```python
from build123d import *

# Parameters (mm, degrees)
SKETCH_1_W                       = 60
SKETCH_1_H                       = 1.5
SM_BASE_FLANGE_1_DEPTH           = 150
SM_EDGE_FLANGE_1_DEPTH           = 150
SM_EDGE_FLANGE_1_2_DEPTH         = 150
SM_EDGE_FLANGE_2_STRIP_W         = 7.4732
SM_EDGE_FLANGE_2_STRIP_H         = 1.5
SM_EDGE_FLANGE_2_STRIP_CUT_DEPTH = 150
SM_EDGE_FLANGE_2_DEPTH           = 150
SKETCH_12_R                      = 2.1
CUT_EXTRUDE_1_DEPTH              = 10
SM_EDGE_FLANGE_3_DEPTH           = 150
SM_EDGE_FLANGE_3_2_DEPTH         = 150
SKETCH_16_R                      = 2.1
CUT_EXTRUDE_2_DEPTH              = 20


# Read off the part's stored shape, not the designer's step: 边线-法兰1, 边线-法兰3
# Sheet-metal steps are written as plain solids
with BuildPart() as part:
    # Sketch 1 → 基体-法兰1 (new body)
    with BuildSketch(Plane.XY):
        with Locations((30, -0.75)):
            Rectangle(SKETCH_1_W, SKETCH_1_H)
    extrude(amount=SM_BASE_FLANGE_1_DEPTH)

    # 边线-法兰1 outline → 边线-法兰1 (cut)
    with BuildSketch(Plane.XY):
        with BuildLine():
            ThreePointArc((54.107469813, 0), (54.399404694, -0.019134423), (54.686344489, -0.076210297))
            Line((54.686344489, -0.076210297), (60, -1.5))
            Line((60, -1.5), (60, 0))
            Line((60, 0), (54.107469813, 0))
        make_face()
    extrude(amount=SM_EDGE_FLANGE_1_DEPTH, mode=Mode.SUBTRACT)

    # Sm Edge Flange 1 2 outline → Sm Edge Flange 1 2 (add)
    with BuildSketch(Plane.XY):
        with BuildLine():
            Line((109.459695887, -14.752685571), (60, -1.5))
            Line((60, -1.5), (54.107469813, -1.5))
            ThreePointArc((54.107469813, -1.5), (54.203615406, -1.506301715), (54.298115921, -1.525099036))
            Line((54.298115921, -1.525099036), (109.071467319, -16.20157431))
            Line((109.071467319, -16.20157431), (109.459695887, -14.752685571))
        make_face()
    extrude(amount=SM_EDGE_FLANGE_1_2_DEPTH)

    # 边线-法兰2 strip (across the edge) → 边线-法兰2 strip cut (cut)
    with BuildSketch(Plane(origin=(0, -1.5, 150), x_dir=(1, 0, 0), z_dir=(0, 0, -1))):
        with Locations((-1.5, -0.75)):
            Rectangle(SM_EDGE_FLANGE_2_STRIP_W, SM_EDGE_FLANGE_2_STRIP_H)
    extrude(amount=SM_EDGE_FLANGE_2_STRIP_CUT_DEPTH, mode=Mode.SUBTRACT)

    # 边线-法兰2 section (across the edge) → 边线-法兰2 (add)
    with BuildSketch(Plane(origin=(0, -1.5, 150), x_dir=(1, 0, 0), z_dir=(0, 0, -1))):
        with BuildLine():
            Line((0, 0.7366), (0, 6.5))
            Line((0, 6.5), (1.5, 6.5))
            Line((1.5, 6.5), (1.5, 0.7366))
            ThreePointArc((1.5, 0.7366), (1.715745145, 0.215745145), (2.2366, 0))
            Line((2.2366, 0), (2.2366, -1.5))
            ThreePointArc((2.2366, -1.5), (0.655084973, -0.844915027), (0, 0.7366))
        make_face()
    extrude(amount=SM_EDGE_FLANGE_2_DEPTH)

    # 草图12 → 切除-拉伸1 (cut)
    with BuildSketch(Plane.ZY):
        with Locations(Location((35, -5, 0), (0, 0, 270))):
            Circle(SKETCH_12_R)
        with Locations(Location((75, -5, 0), (0, 0, 270))):
            Circle(SKETCH_12_R)
        with Locations(Location((115, -5, 0), (0, 0, 270))):
            Circle(SKETCH_12_R)
    extrude(amount=-CUT_EXTRUDE_1_DEPTH, mode=Mode.SUBTRACT)

    # 边线-法兰3 outline → 边线-法兰3 (cut)
    with BuildSketch(Plane.XY):
        with BuildLine():
            ThreePointArc((107.413741996, -14.204473878), (108.55784048, -14.938769949), (109.065378631, -16.199942851))
            Line((109.065378631, -16.199942851), (109.071467319, -16.20157431))
            Line((109.071467319, -16.20157431), (109.459695887, -14.752685571))
            Line((109.459695887, -14.752685571), (107.413741996, -14.204473878))
        make_face()
    extrude(amount=SM_EDGE_FLANGE_3_DEPTH, mode=Mode.SUBTRACT)

    # Sm Edge Flange 3 2 outline → Sm Edge Flange 3 2 (add)
    with BuildSketch(Plane.XY):
        with BuildLine():
            Line((109.071467319, -25.64866004), (109.071467319, -16.364863581))
            ThreePointArc((109.071467319, -16.364863581), (109.069944629, -16.282347038), (109.065378631, -16.199942851))
            Line((109.065378631, -16.199942851), (107.025513428, -15.653362617))
            ThreePointArc((107.025513428, -15.653362617), (107.41925139, -15.916449912), (107.571467319, -16.364863581))
            Line((107.571467319, -16.364863581), (107.571467319, -25.64866004))
            Line((107.571467319, -25.64866004), (109.071467319, -25.64866004))
        make_face()
    extrude(amount=SM_EDGE_FLANGE_3_2_DEPTH)

    # 草图16 → 切除-拉伸2 (cut)
    with BuildSketch(Plane.ZY.offset(-107.571467319)):
        with Locations(Location((35, -21.00676181, 0), (0, 0, 270))):
            Circle(SKETCH_16_R)
        with Locations(Location((75, -21.00676181, 0), (0, 0, 270))):
            Circle(SKETCH_16_R)
        with Locations(Location((115, -21.00676181, 0), (0, 0, 90))):
            Circle(SKETCH_16_R)
    extrude(amount=-CUT_EXTRUDE_2_DEPTH, mode=Mode.SUBTRACT)


solid = part.part
```
The listing builds one solid part. Answer for the finished solid, in the listing's coordinates (mm). A direction names the side the tool comes from. Round coordinates to 2 decimals unless told otherwise and drop trailing zeros. Loops run counter-clockwise (first coordinate to the right, second up) from the corner with the lowest first, then second, coordinate; pieces in that order, holes last.
1) For faces 4 (the face through (108.31, -19.34, 33.72)), 5 (the face through (107.571, -18.9, 74)), 6 (the face through (28, -1.5, 74)), 7 (the face through (0.74, -3.452, 76.419)), 8 (the face through (0, -7, 76.05)), determine the directions among +Z, -Z, +X, -X, +Y, -Y from which every point of the face is accessible in a straight line to the end or side of a thin tool.
Outcome:
face 4: +X, -X
face 5: +Z, -Z, -X, -Y
face 6: +Z, -Z, -Y
face 7: -X
face 8: +Z, -Z, -X, +Y, -Y
2) For a pull along Y with two mould halves and no side action, classify faces 1 (the face through (1.5, -7.1, 76)), 2 (the face through (108.31, -19.34, 73.72)), 3 (the face through (80.29, -8.49, 73.95)) as released by +Y, released by -Y, zero draft, split by the parting line, or undercut.
Outcome:
face 1: zero draft
face 2: undercut
face 3: released by -Y
3) Consider line 1 (Z direction, x = 1.15, y = -5); line 2 (Y direction, x = 48.5, z = 43.5); line 3 (X direction, y = -18.75, z = 110). Determine where each line is inside the solid, lowest interval first.
Outcome:
line 1: z = 0 to 32.9, 37.1 to 72.9, 77.1 to 112.9, 117.1 to 150
line 2: y = -1.5 to 0
line 3: x = 107.57 to 109.07
4) A cutting plane is placed at A-A on z = 75. Determine the outline of the cut face in (x, y).
Outcome:
outline: (0, -8) - (1.5, -8) - (1.5, -7.1) - (0, -7.1) - close; (0, -2.9) - (1.5, -2.9) - (1.5, -2.24) arc R0.74 cw to (2.24, -1.5) - (54.11, -1.5) arc R0.74 cw to (54.3, -1.53) - (107.03, -15.65) arc R0.74 cw to (107.57, -16.36) - (107.57, -18.91) - (109.07, -18.91) - (109.07, -16.36) arc R2.24 ccw to (107.41, -14.2) - (54.69, -0.08) arc R2.24 ccw to (54.11, 0) - (2.24, 0) arc R2.24 ccw to (0, -2.24) - close; (107.57, -25.65) - (109.07, -25.65) - (109.07, -23.11) - (107.57, -23.11) - close
5) Given P1, Ø1, axis at x = 64.5, z = 52, coming from the -Y side; P2, Ø5, axis at y = -21.01, z = 35, coming from the -X side; P3, Ø0.8, axis at x = 0.5, z = 99, coming from the -Y side, each flat-ended and moving along its own axis, determine where each tip first touches the part or whether it passes through.
Outcome:
P1: stops at y = -4.39
P2: stops at x = 107.57
P3: stops at y = -8
6) A cutting plane is placed at D-D on x = 42. Determine the outline of the cut face in (y, z), plus the area to 3 significant figures.
Outcome:
outline: (-1.5, 0) - (0, 0) - (0, 150) - (-1.5, 150) - close
area: 225 mm2
7) A cutting plane is placed at C-C on z = 11. Determine the outline of the cut face in (x, y), plus the area to 3 significant figures.
Outcome:
outline: (0, -8) - (1.5, -8) - (1.5, -2.24) arc R0.74 cw to (2.24, -1.5) - (54.11, -1.5) arc R0.74 cw to (54.3, -1.53) - (107.03, -15.65) arc R0.74 cw to (107.57, -16.36) - (107.57, -25.65) - (109.07, -25.65) - (109.07, -16.36) arc R2.24 ccw to (107.41, -14.2) - (54.69, -0.08) arc R2.24 ccw to (54.11, 0) - (2.24, 0) arc R2.24 ccw to (0, -2.24) - close
area: 189 mm2
8) A cutting plane is placed at B-B on y = -5. Determine the outline of the cut face in (x, z).
Outcome:
outline: (0, 0) - (1.5, 0) - (1.5, 32.9) - (0, 32.9) - close; (0, 37.1) - (1.5, 37.1) - (1.5, 72.9) - (0, 72.9) - close; (0, 77.1) - (1.5, 77.1) - (1.5, 112.9) - (0, 112.9) - close; (0, 117.1) - (1.5, 117.1) - (1.5, 150) - (0, 150) - close; (67.27, 0) - (73.06, 0) - (73.06, 150) - (67.27, 150) - close
